Geometry: final body of the model. Coordinates: model frame, mm. A direction names the side the tool comes from. Give positions to 0.01 mm unless a question says otherwise; leave off trailing zeros. Loops run counter-clockwise (first coordinate to the right, second up) from the corner with the lowest first, then second, coordinate; pieces in that order, holes last. Notation, with made-up numbers: (72, 34) -> (78, 34) arc R26 cw to (78, 70) -> close; hole circle Ø6 at (27.25, 6). An arc over 180 degrees is marked (long way). Answer in a Markdown table with one row per item. Add a question column.
1) Draft query along Z for faces 1 (the flat face through (33, 36, 26.227)), 2 (the flat face through (45, 36, 30)), 3 (the flat face through (-38.822, 35.916, 39.873)). Return one class per face: +Z half, -Z half, draft (parallel to the pull), parting line (faces both ways), or undercut.
2) Section query C-C (y = 32). Return the cut outline in (x, z).
3) Section query B-B (x = -2). Return the cut outline in (y, z), plus the area to 3 significant figures.
4) Access query for faces 4 (the flat face through (30, 30, 36)), 5 (the flat face through (-1, 42, 21)), 6 (the flat face through (7.5, 17, -86)), 7 (the flat face through (-30, 30, 36)). Directions: +Z, -Z, +X, -X, +Y, -Y. A direction counts if a zero-diameter tool reaches every point of the face in a straight line with its end or side. Return the directions, or none.
5) Line query: line 1 (Z direction, x = 23, y = 38.5); line 2 (Y direction, x = 9, z = 12); line 3 (Y direction, x = 39, z = 16). Output: solid intervals per line, ascending. Write a range as from..to.
6) Section query A-A (x = -27.5). Return the cut outline in (y, z), plus the area to 3 significant figures.
7) First-contact query: P1, Ø18, axis at y = 18, z = -97, coming from the +X side; P2, Ø20, axis at x = -5.5, z = -27, coming from the +Y side; P3, Ø6, axis at y = 14, z = 37.5, coming from the -X side; P4, Ø1, axis at x = -22, z = -18.5, coming from the +Y side. Flat tips, straight axial feed; report the tip coordinate or a pass-through.
8) Section query D-D (z = 11). Return the cut outline in (x, y).
```python
from build123d import *

# Parameters (mm, degrees)
SKETCH1_W           = 95
SKETCH1_H           = 30
BOSS_EXTRUDE1_DEPTH = 40
BOSS_EXTRUDE2_DEPTH = 12
SKETCH4_R           = 5
CUT_EXTRUDE1_DEPTH  = 87.62461911
SKETCH6_R           = 30
SKETCH6_R_2         = 12.5
BOSS_EXTRUDE3_DEPTH = 7.5


with BuildPart() as part:
    # Sketch1 → Boss-Extrude1 (new body)
    with BuildSketch(Plane(origin=(0, 0, 0), x_dir=(0, 0, -1), z_dir=(1, 0, 0))):
        with Locations((1.273195876, 15)):
            Rectangle(SKETCH1_W, SKETCH1_H)
    extrude(amount=-BOSS_EXTRUDE1_DEPTH)

    # Sketch3 → Boss-Extrude2 (add)
    with BuildSketch(Plane(origin=(0, 30, 0), x_dir=(1, 0, 0), z_dir=(0, 1, 0))):
        with BuildLine():
            ThreePointArc((0, -26.226804124), (-5, -21.226804124), (0, -16.226804124))
            Line((0, -16.226804124), (0, 3.773195876))
            Line((0, 3.773195876), (-40, 3.741487841))
            Line((-40, 3.741487841), (-40, -16.226804124))
            ThreePointArc((-40, -16.226804124), (-35, -21.226804124), (-40, -26.226804124))
            Line((-40, -26.226804124), (-40, -46.226804124))
            Line((-40, -46.226804124), (0, -46.226804124))
            Line((0, -46.226804124), (0, -26.226804124))
        make_face()
        Polygon((-52.468291965, -46.226804124), (-40, -46.226804124), (-40, -26.226804124), (-65, -26.226804124), (-65, -33.695096088), align=None)
        Polygon((-40, -16.226804124), (-40, 3.741487841), (-52.5, 3.741487841), (-65, -8.758512159), (-65, -16.226804124), align=None)
        Polygon((25, -26.226804124), (0, -26.226804124), (0, -46.226804124), (12.468291965, -46.226804124), (25, -33.695096088), align=None)
        Polygon((0, 3.773195876), (0, -16.226804124), (25, -16.226804124), (25, -8.758512159), (12.468291965, 3.773195876), align=None)
    extrude(amount=BOSS_EXTRUDE2_DEPTH)

    # Sketch4 → Cut-Extrude1 (cut, through all)
    with BuildSketch(Plane(origin=(0, 30, 0), x_dir=(1, 0, 0), z_dir=(0, 1, 0))):
        with Locations((0, -21.226804124)):
            Circle(SKETCH4_R)
        with Locations((-40, -21.226804124)):
            Circle(SKETCH4_R)
    extrude(amount=-CUT_EXTRUDE1_DEPTH, mode=Mode.SUBTRACT)


with BuildPart() as part_1:
    # Body-Move_Copy1: moved
    add(part.part.moved(Location((20, 0, 0))))

    # Sketch6 → Boss-Extrude3 (add, symmetric)
    # profile 1 of 2: a face of its own
    with BuildSketch(Plane(origin=(0, 0, 0), x_dir=(0, 0, -1), z_dir=(1, 0, 0))):
        with BuildLine():
            Line((63.773195876, 30), (48.773195876, 30))
            Line((48.773195876, 30), (48.773195876, 0))
            Line((48.773195876, 0), (93.773195876, 0))
            ThreePointArc((93.773195876, 0), (72.559992441, 8.786796564), (63.773195876, 30))
        make_face()
    # profile 2 of 2: a face of its own
    with BuildSketch(Plane(origin=(0, 0, 0), x_dir=(0, 0, -1), z_dir=(1, 0, 0))):
        with Locations((93.773195876, 30)):
            Circle(SKETCH6_R)
        with Locations((93.773195876, 30)):
            Circle(SKETCH6_R_2, mode=Mode.SUBTRACT)
    extrude(amount=BOSS_EXTRUDE3_DEPTH, both=True)


solid = part_1.part
```
Evaluation:
| question | item | result |
|---|---|---|
| 1 | face 1 | undercut |
| 1 | face 2 | draft |
| 1 | face 3 | +Z half |
| 2 | outline | (-45, 8.76) -> (-32.5, -3.74) -> (-20, -3.74) -> (20, -3.77) -> (32.47, -3.77) -> (45, 8.76) -> (45, 16.23) -> (20, 16.23) arc R5 cw to (20, 26.23) -> (45, 26.23) -> (45, 33.7) -> (32.47, 46.23) -> (-32.47, 46.23) -> (-45, 33.7) -> (-45, 26.23) -> (-20, 26.23) arc R5 cw to (-20, 16.23) -> (-45, 16.23) -> close; (-7.5, -123.71) -> (7.5, -123.71) -> (7.5, -106.11) -> (-7.5, -106.11) -> close; (-7.5, -81.43) -> (7.5, -81.43) -> (7.5, -63.84) -> (-7.5, -63.84) -> close |
| 3 | outline | (0, -93.77) arc R30 ccw (long way) to (30, -63.77) -> (30, -3.76) -> (42, -3.76) -> (42, 46.23) -> (0, 46.23) -> close; hole circle Ø25 at (30, -93.77) |
| 3 | area | 6,430 mm² |
| 4 | face 4 | +Z, -Z, +X, -Y |
| 4 | face 5 | +Z, +X, -X, +Y |
| 4 | face 6 | -Z, +X, +Y, -Y |
| 4 | face 7 | +Z, -Z, -X, -Y |
| 5 | line 1 | -3.77..16.23, 26.23..46.23 |
| 5 | line 2 | 0..42 |
| 5 | line 3 | 30..42 |
| 6 | outline | (30, -3.74) -> (42, -3.74) -> (42, 16.23) -> (30, 16.23) -> close; (30, 26.23) -> (42, 26.23) -> (42, 46.23) -> (30, 46.23) -> close |
| 6 | area | 480 mm² |
| 7 | P1 | x = 7.5 |
| 7 | P2 | y = 30 |
| 7 | P3 | x = -20 |
| 7 | P4 | through |
| 8 | outline | (-45, 30) -> (-20, 30) -> (-20, 0) -> (20, 0) -> (20, 30) -> (45, 30) -> (45, 42) -> (-45, 42) -> close |
